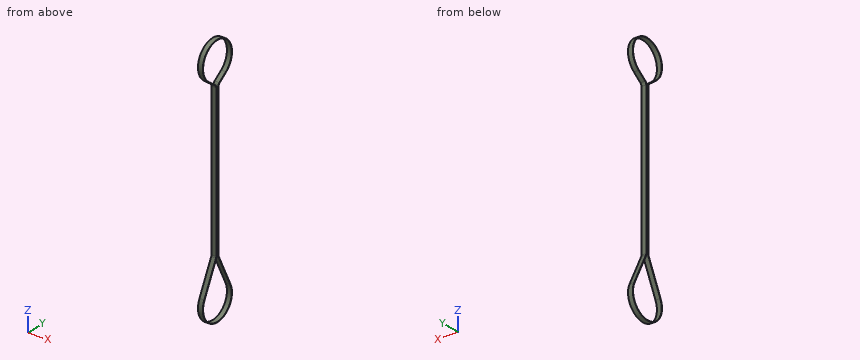
Autodesk Inventor part; units mm, degrees
ref_plane "YZ Plane" through (0, 0, 0) normal (1, 0, 0) x (0, 1, 0)
ref_plane "XZ Plane" through (0, 0, 0) normal (0, 1, 0) x (-1, 0, 0)
ref_plane "XY Plane" through (0, 0, 0) normal (0, 0, 1) x (1, 0, 0)
sketch "スケッチ1" plane through (0, 0, 0) normal (1, 0, 0) x (0, 1, 0)
  arc A0 (23.0723, -31.0387) -> (-23.0723, -31.0387) centre (0, 0) ccw
  arc A1 (-34.7971, -433.1214) -> (34.7971, -433.1214) centre (0, -450) ccw
  arc A2 (-2.581, -50) -> (-5.574, -44.0458) centre (-10, -50) ccw
  line L0 (-5.574, -44.0458) -> (-23.0723, -31.0387)
  line L1 (23.0723, -31.0387) -> (5.574, -44.0458)
  line L2 (34.7971, -433.1214) -> (3.3248, -368.2378)
  line L3 (-34.7971, -433.1214) -> (-3.3248, -368.2378)
  arc A3 (5.574, -44.0458) -> (2.581, -50) centre (10, -50) ccw
  arc A4 (2.581, -365) -> (3.3248, -368.2378) centre (10, -365) ccw
  arc A5 (-3.3248, -368.2378) -> (-2.581, -365) centre (-10, -365) ccw
  line L4 (-2.581, -50) -> (-2.581, -365)
  line L5 (2.581, -365) -> (2.581, -50)
  line L6 (5.824, -44.3821) -> (23.3222, -31.3749)
  arc A6 (23.3222, -31.3749) -> (-23.3222, -31.3749) centre (0, 0) ccw
  line L7 (-23.3222, -31.3749) -> (-5.824, -44.3821)
  arc A7 (-3, -50) -> (-5.824, -44.3821) centre (-10, -50) ccw
  line L8 (-3, -50) -> (-3, -365)
  arc A8 (-3.7018, -368.055) -> (-3, -365) centre (-10, -365) ccw
  line L9 (-3.7018, -368.055) -> (-35.1741, -432.9385)
  arc A9 (-35.1741, -432.9385) -> (35.1741, -432.9385) centre (0, -450) ccw
  line L10 (35.1741, -432.9385) -> (3.7018, -368.055)
  arc A10 (3, -365) -> (3.7018, -368.055) centre (10, -365) ccw
  line L11 (3, -365) -> (3, -50)
  arc A11 (5.824, -44.3821) -> (3, -50) centre (10, -50) ccw
  arc A12 (5.3467, -43.74) -> (2.2, -50) centre (10, -50) ccw
  line L12 (5.3467, -43.74) -> (22.845, -30.7329)
  arc A13 (22.845, -30.7329) -> (-22.845, -30.7329) centre (0, 0) ccw
  line L13 (-22.845, -30.7329) -> (-5.3467, -43.74)
  arc A14 (-2.2, -50) -> (-5.3467, -43.74) centre (-10, -50) ccw
  line L14 (-2.2, -50) -> (-2.2, -365)
  arc A15 (-2.982, -368.4041) -> (-2.2, -365) centre (-10, -365) ccw
  line L15 (-2.982, -368.4041) -> (-34.4543, -433.2876)
  arc A16 (-34.4543, -433.2876) -> (34.4543, -433.2876) centre (0, -450) ccw
  line L16 (34.4543, -433.2876) -> (2.982, -368.4041)
  arc A17 (2.2, -365) -> (2.982, -368.4041) centre (10, -365) ccw
  line L17 (2.2, -365) -> (2.2, -50)
  dimension "d0" = 77.3493
  dimension "d1" = 77.3493
  dimension "d2" = 450
  dimension "d39" = 0.419
  dimension "d40" = 0.8
  dimension "d41" = 7
  dimension "d42" = 7
  dimension "d43" = 7
  dimension "d44" = 7
  dimension "d45" = 10
  dimension "d46" = 10
  dimension "d47" = 85
  dimension "d48" = 50
extrude "押し出し1" add sketch "スケッチ1" along normal mid plane 10 contours L1 A3 L5 A4 L2 A1 L3 A5 L4 A2 L0 A0 | A11 L11 A10 L10 A9 L9 A8 L8 A7 L7 A6 L6
equation "\"d0\" = d1"
equation "\"d41\" = d43"
equation "\"d43\" = d44"
equation "\"d44\" = d42"
properties part number "scara-belt1" material "ゴム"
Can you work these out from the model? Positions are in its coordinate system, mm. Give positions to 0.01 mm unless a question says otherwise; leave off trailing zeros. Order: outer loops, then holes, each group sorted by start corner. A loop starts at its lowest first (then second) coordinate and runs counter-clockwise, first axis right, second up. Notation, with made-up numbers: M -32,-20 L -10,-20 A20 ccw -10,11 Z; hole C 29,74 d7. An arc over 180 degrees is marked long. One line per item, written item: value.
Item 1: Please list where these lines run through material, in increasing order: line 1 (Z direction, x = 1.75, y = 0); line 2 (Z direction, x = 1.5, y = 14); line 3 (Y direction, x = 3, z = -148).
Verdict:
line 1: -489.09 to -488.29, 38.29 to 39.09
line 2: -486.5 to -485.64, -391.12 to -389.29, -38.3 to -37.31, 35.64 to 36.5
line 3: -3 to -2.2, 2.2 to 3
Item 2: If we section it at B-B on x = -1.25: Write out the boundary of the cut face in (y, z) (1 decimal).
Verdict:
outline: M -35.2,-432.9 A39.1 ccw long 35.2,-432.9 L 3.7,-368.1 A7 cw 3,-365 L 3,-50 A7 cw 5.8,-44.4 L 23.3,-31.4 A39.1 ccw long -23.3,-31.4 L -5.8,-44.4 A7 cw -3,-50 L -3,-365 A7 cw -3.7,-368.1 Z; hole M -34.5,-433.3 A38.3 ccw long 34.5,-433.3 L 3,-368.4 A7.8 cw 2.2,-365 L 2.2,-50 A7.8 cw 5.3,-43.7 L 22.8,-30.7 A38.3 ccw long -22.8,-30.7 L -5.3,-43.7 A7.8 cw -2.2,-50 L -2.2,-365 A7.8 cw -3,-368.4 Z
Item 3: If we section it at A-A on z = -450: Write out the boundary of the cut face in (x, y).
Verdict:
outline: M -5,-39.09 L 5,-39.09 L 5,-38.29 L -5,-38.29 Z; M -5,38.29 L 5,38.29 L 5,39.09 L -5,39.09 Z
Item 4: If we section it at C-C on y = -18: Write out the boundary of the cut face in (x, z).
Verdict:
outline: M -5,-484.7 L 5,-484.7 L 5,-483.8 L -5,-483.8 Z; M -5,-399.37 L 5,-399.37 L 5,-397.53 L -5,-397.53 Z; M -5,-35.33 L 5,-35.33 L 5,-34.33 L -5,-34.33 Z; M -5,33.8 L 5,33.8 L 5,34.7 L -5,34.7 Z
Item 5: For pin 1 (1.5 mm diameter, centred on x = 3, z = -43.5, fed in from -Y); pin 2 (2 mm diameter, centred on x = 2, z = -45, fed in from -Y); pin 3 (6 mm diameter, centred on x = 0, z = -152, fed in from -Y), each with a flat end and sliding along its axis, tell me the tip position at first contact or that it passes through.
Verdict:
pin 1: y = -8.02
pin 2: y = -6.34
pin 3: y = -3
